Geometry: final body of the model. Coordinates: model frame, mm. Round coordinates to 2 decimals unless told otherwise and drop trailing zeros. Write each loop counter-clockwise with the first axis right and the second up, starting at its lowest first coordinate (ties: lowest second). Pieces come first, ordered by that corner, then holes. Notation, with made-up numbers: M -8.75,55 L 29.25,55 A21 cw 29.25,81 Z; hole C -15,-17 d10. An arc over 180 degrees is marked long. Answer as CSV lines item,"result". Start each with the question number.
Q1. Section query B-B on x = 344.5. Output: boundary loops of the cut face in (y, z).
Q2. Section query A-A on z = 45.5. Output: boundary loops of the cut face in (x, y), and give its area (3 significant figures).
Q3. First-contact query: pin 1 (1.9 mm diameter, centred on x = 223, y = -3, fed in from -Z); pin 2 (3 mm diameter, centred on y = -3.5, z = 3.5, fed in from -X); pin 3 (3 mm diameter, centred on x = 267, z = 55.5, fed in from +Y); pin 4 (1.9 mm diameter, centred on y = -4, z = 68, fed in from +X). Flat tips, straight axial feed; report the tip coordinate or a pass-through.
Q4. Ray query, probe 1 along X at (y, z) = (-3, 6); probe 2 along X at (y, z) = (-0.25, 65.5); probe 3 along Z at (x, y) = (228.5, -0.5). Return the intervals inside material, ascending.
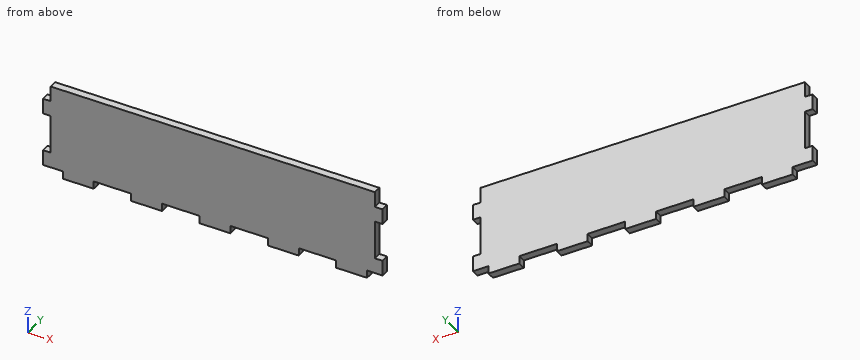
```python
from build123d import *

# Parameters (mm, degrees)
F0_W     = 444.5
F0_H     = 76.2
F1_DEPTH = 6.35
F2_W     = 6.35
F2_H     = 6.35
F2_H_2   = 12.7
F2_H_3   = 31.75
F3_DEPTH = 6.35
F4_W     = 30.842857
F4_H     = 6.35
F4_W_2   = 30.842858
F4_W_3   = 6.35
F5_DEPTH = 6.351
F6_W     = 165.1
F6_H     = 76.2
F7_DEPTH = 6.351
F8_W     = 6.35
F8_H     = 12.7
F8_H_2   = 31.75
F9_DEPTH = 6.351


with BuildPart() as f1:
    # F0 (on Front) → F1 (new body)
    with BuildSketch(Plane.XZ):
        with Locations((222.25, 38.1)):
            Rectangle(F0_W, F0_H)
    extrude(amount=F1_DEPTH)

    # F2 (on face) → F3 (cut, through all)
    with BuildSketch(Plane.XZ.offset(6.35)):
        with Locations((3.175, 3.175)):
            Rectangle(F2_W, F2_H)
        with Locations((3.175, 69.85)):
            Rectangle(F2_W, F2_H_2)
        with Locations((3.175, 34.925)):
            Rectangle(F2_W, F2_H_3)
        with Locations((441.325, 3.175)):
            Rectangle(F2_W, F2_H)
        with Locations((441.325, 34.925)):
            Rectangle(F2_W, F2_H_3)
        with Locations((441.325, 69.85)):
            Rectangle(F2_W, F2_H_2)
    extrude(amount=-F3_DEPTH, mode=Mode.SUBTRACT)

    # F4 (on face) → F5 (cut, through all)
    with BuildSketch(Plane.XZ.offset(6.35)):
        with Locations((53.521428, 3.175)):
            Rectangle(F4_W, F4_H)
        with Locations((109.764285, 3.175)):
            Rectangle(F4_W, F4_H)
        with Locations((166.007142, 3.175)):
            Rectangle(F4_W, F4_H)
        with Locations((222.25, 3.175)):
            Rectangle(F4_W_2, F4_H)
        with Locations((278.492858, 3.175)):
            Rectangle(F4_W, F4_H)
        with Locations((334.735714, 3.175)):
            Rectangle(F4_W, F4_H)
        with Locations((390.978571, 3.175)):
            Rectangle(F4_W, F4_H)
        with Locations((9.525, 3.175)):
            Rectangle(F4_W_3, F4_H)
        with Locations((434.975, 3.175)):
            Rectangle(F4_W_3, F4_H)
    extrude(amount=-F5_DEPTH, mode=Mode.SUBTRACT)

    # F6 (on face) → F7 (cut, through all)
    with BuildSketch(Plane.XZ.offset(6.35)):
        with Locations((82.55, 38.1)):
            Rectangle(F6_W, F6_H)
    extrude(amount=-F7_DEPTH, mode=Mode.SUBTRACT)

    # F8 (on face) → F9 (cut, through all)
    with BuildSketch(Plane.XZ.offset(6.35)):
        with Locations((168.275, 69.85)):
            Rectangle(F8_W, F8_H)
        with Locations((168.275, 34.925)):
            Rectangle(F8_W, F8_H_2)
    extrude(amount=-F9_DEPTH, mode=Mode.SUBTRACT)


solid = f1.part
```
Entries:
1,outline,"M -6.35,6.35 L 0,6.35 L 0,76.2 L -6.35,76.2 Z"
2,outline,"M 171.45,-6.35 L 438.15,-6.35 L 438.15,0 L 171.45,0 Z"
2,area,"1,690 mm^2"
3,pin 1,"stops at z = 6.35"
3,pin 2,"stops at x = 181.43"
3,pin 3,"stops at y = 0"
3,pin 4,"stops at x = 438.15"
4,probe 1,"x = 181.43 to 206.83, 237.67 to 263.07, 293.91 to 319.31, 350.16 to 375.56, 406.4 to 431.8"
4,probe 2,"x = 171.45 to 438.15"
4,probe 3,"z = 6.35 to 76.2"
